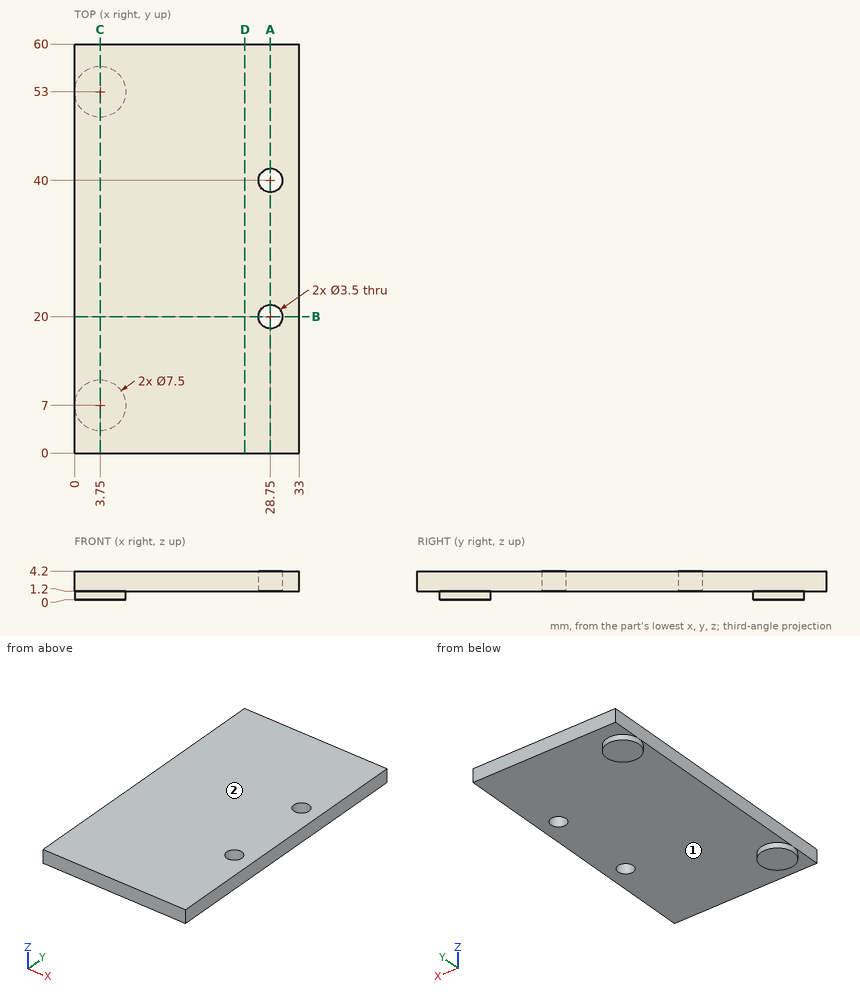
Drawing for the job (mm, zero at the part's lowest x, y, z). Coordinates: 2 decimals unless noted, no trailing zeros. Loops run counter-clockwise (first coordinate to the right, second up) from the corner with the lowest first, then second, coordinate; pieces in that order, holes last. Notation, with made-up numbers: (68, -25.75) - (104, -25.75) arc R15 ccw to (104, -10.75) - close; hole circle Ø7 at (78.5, 53.5). An arc over 180 degrees is marked (long way). Use CSV: the item, a comma, the result in double quotes. Start each with the question number.
Q1. Cut at C-C, the plane x = 3.75. List the corners of the cut face in (y, z).
Q2. Cut at A-A, the plane x = 28.75. List the corners of the cut face in (y, z), then the cut area to 3 significant figures.
Q3. Probe probe 1 along Y at (x, z) = (28.75, 2.6); probe 2 along Z at (x, y) = (9, 50); probe 3 along Y at (x, z) = (5.5, 1.05). List the from-to ranges inside material, lowest first. Write a range as from..to.
Q4. Cut at D-D, the plane x = 25. List the corners of the cut face in (y, z).
Q5. Drop flat-ended pins along their axis: P1, Ø3, axis at x = 28.75, y = 40, coming from the -Z side; P2, Ø10, axis at x = 12.5, y = 16, coming from the -Z side. Give the stop position or say it passes through.
Q6. Cut at B-B, the plane y = 20. List the corners of the cut face in (x, z), then the cut area to 3 significant figures.
Q7. Two-plate mould, pull along Y, no slides. Class the marked faces 1 and 2: +Y half, -Y half, draft (parallel to the pull), parting line (faces both ways), or undercut.
Here are the results:
1,outline,"(0, 1.2) - (3.25, 1.2) - (3.25, 0) - (10.75, 0) - (10.75, 1.2) - (49.25, 1.2) - (49.25, 0) - (56.75, 0) - (56.75, 1.2) - (60, 1.2) - (60, 4.2) - (0, 4.2) - close"
2,outline,"(0, 1.2) - (18.25, 1.2) - (18.25, 4.2) - (0, 4.2) - close; (21.75, 1.2) - (38.25, 1.2) - (38.25, 4.2) - (21.75, 4.2) - close; (41.75, 1.2) - (60, 1.2) - (60, 4.2) - (41.75, 4.2) - close"
2,area,"159 mm2"
3,probe 1,"0..18.25, 21.75..38.25, 41.75..60"
3,probe 2,"1.2..4.2"
3,probe 3,"3.68..10.32, 49.68..56.32"
4,outline,"(0, 1.2) - (60, 1.2) - (60, 4.2) - (0, 4.2) - close"
5,P1,"through"
5,P2,"z = 1.2"
6,outline,"(0, 1.2) - (27, 1.2) - (27, 4.2) - (0, 4.2) - close; (30.5, 1.2) - (33, 1.2) - (33, 4.2) - (30.5, 4.2) - close"
6,area,"88.5 mm2"
7,face 1,"undercut"
7,face 2,"draft"
